Autodesk Inventor part; units mm, degrees
ref_plane "YZ Plane" through (0, 0, 0) normal (1, 0, 0) x (0, 1, 0)
ref_plane "XZ Plane" through (0, 0, 0) normal (0, 1, 0) x (-1, 0, 0)
ref_plane "XY Plane" through (0, 0, 0) normal (0, 0, 1) x (1, 0, 0)
sketch "Sketch1" plane through (0, 0, 0) normal (0, 0, 1) x (1, 0, 0)
  circle A0 centre (0, 0) radius 2.4 construction
  line L0 (-0.8, 2.2627) -> (-0.8, 0.8)
  line L1 (-0.8, 0.8) -> (-2.2627, 0.8)
  line L2 (-2.2627, -0.8) -> (-0.8, -0.8)
  line L3 (-0.8, -0.8) -> (-0.8, -2.2627)
  line L4 (0.8, -2.2627) -> (0.8, -0.8)
  line L5 (0.8, -0.8) -> (2.2627, -0.8)
  line L6 (2.2627, 0.8) -> (0.8, 0.8)
  line L7 (0.8, 0.8) -> (0.8, 2.2627)
  arc A1 (0.8, 2.2627) -> (-0.8, 2.2627) centre (0, 0) ccw
  arc A2 (-2.2627, 0.8) -> (-2.2627, -0.8) centre (0, 0) ccw
  arc A3 (-0.8, -2.2627) -> (0.8, -2.2627) centre (0, 0) ccw
  arc A4 (2.2627, -0.8) -> (2.2627, 0.8) centre (0, 0) ccw
  dimension "d0" = 4.8
  dimension "d1" = 1.6
extrude "Extrusion1" add sketch "Sketch1" along normal mid plane 24
fillet "Fillet1" radius 0.4 8 edges at (0, 2.4, 12) (-2.4, 0, 12) (0, -2.4, 12) (2.4, 0, 12) (2.4, 0, -12) (0, 2.4, -12) (-2.4, 0, -12) (0, -2.4, -12)
equation "\"d0\" = kd"
equation "\"d1\" = axlet"
equation "\"d2\" = 3 * lu"
equation "\"d4\" = tf"
properties part number "4519-Yellow" material "ABS Plastic"
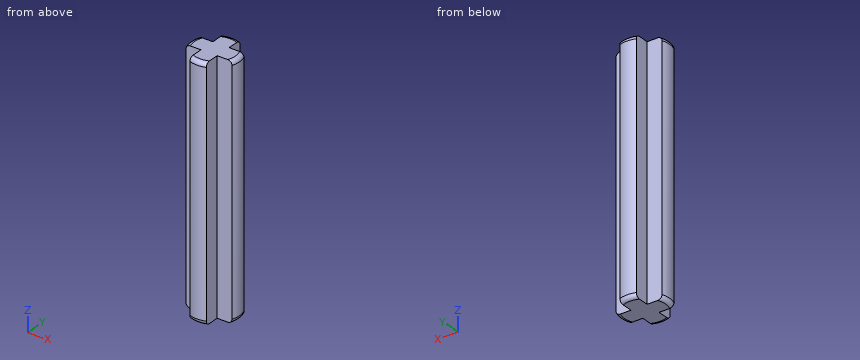
Here's how the part is built. I have some questions about the finished solid (model axes, mm). Coordinates: 2 decimals unless noted, no trailing zeros. Loops run counter-clockwise (first coordinate to the right, second up) from the corner with the lowest first, then second, coordinate; pieces in that order, holes last. Notation, with made-up numbers: M 20,-8 L 72,-8 A29 cw 72,14 Z; hole C -2.75,-39.5 d11. An arc over 180 degrees is marked long. One line per item, written item: value.
1. Imagine slicing it at B-B (y = -1.45). List the corners of the cut face in (x, z) for me.
Geometry says:
outline: M -0.8,-12 L 0.8,-12 L 0.8,12 L -0.8,12 Z
2. Imagine slicing it at A-A (z = 4). List the corners of the cut face in (x, y) for me.
Geometry says:
outline: M -2.26,-0.8 L -0.8,-0.8 L -0.8,-2.26 A2.4 ccw 0.8,-2.26 L 0.8,-0.8 L 2.26,-0.8 A2.4 ccw 2.26,0.8 L 0.8,0.8 L 0.8,2.26 A2.4 ccw -0.8,2.26 L -0.8,0.8 L -2.26,0.8 A2.4 ccw Z
3. Will these pins go through, and if not, where does the flat tip stop? pin 1 Ø1.6 at (x, z) = (1.5, -2) entering from +Y; pin 2 Ø1.2 at (x, z) = (-2, 5.5) entering from -Y; pin 3 Ø1.2 at (y, z) = (-1.5, 4.5) entering from +X.
Geometry says:
pin 1: stops at y = 2.3
pin 2: stops at y = -0.8
pin 3: stops at x = 0.8
4. Please list where these lines run through material, in increasing order: probe 1 along Y at (x, z) = (0.85, 0.5); probe 2 along X at (y, z) = (0.1, -1.75).
Geometry says:
probe 1: y = -0.8 to 0.8
probe 2: x = -2.4 to 2.4
